For this review, take the finished solid that the model builds, in its own axes (mm). Face numbers are marked on the shaded views. A direction names the side the tool comes from. Give positions to 0.01 mm unless a question says otherwise; leave off trailing zeros. Loops run counter-clockwise (first coordinate to the right, second up) from the corner with the lowest first, then second, coordinate; pieces in that order, holes last. Notation, with made-up numbers: (32.5, -21) -> (86.5, -21) arc R33 ccw to (86.5, 8) -> close; hole circle Ø5 at (-32.75, 43). An arc over 180 degrees is marked (long way). Answer as CSV lines item,"result". Start each with the question number.
Item 1: Add section C-C on z = 2. State the section outline as (x, y) points, plus the area to 3 significant figures.
Item 2: Add section B-B on z = -51.5. State the section outline as (x, y) points, plus the area to 3 significant figures.
Item 3: For L1, parallel to Z at x = 6.3, y = 0; L2, parallel to Y at x = 2, z = -18; L3, parallel to X at y = -7, z = 8.5, list the stretches that pass through material, from the lowest coordinate up. Write a range as from..to.
Item 4: Add section A-A on x = -1.25. State the section outline as (y, z) points, plus the area to 3 significant figures.
Item 5: Machinability: for the marked faces 1 and 2, which of the approach directions +Z, -Z, +X, -X, +Y, -Y give a long, thin tool a straight path to every point of the face, cutting with its end or side? Answer none if there is none.
Item 6: The part is to be moulded in two halves that separate along X. For the marked faces 3, 4 and 5, say which applies: +X half, -X half, draft (parallel to the pull), parting line (faces both ways), or undercut.
Item 7: Clearance check with flat-ended pins moving along their axes: P1, Ø3.5, axis at x = 2, y = 3, coming from the -Z side; P2, Ø6, axis at x = -0.5, z = -47.5, coming from the +Y side; P3, Ø10, axis at y = -10, z = -10.5, coming from the +X side; P4, Ø1.5, axis at y = -9.5, z = -15, coming from the -X side. State where each tip first meets the part, or that it passes through.
```python
from build123d import *

# Parameters (mm, degrees)
SKETCH1_W           = 11.7
SKETCH1_H           = 18.2
SKETCH1_W_2         = 6.2
SKETCH1_H_2         = 15.2
BOSS_EXTRUDE1_DEPTH = 12
SKETCH4_R           = 2.55
CUT_EXTRUDE1_DEPTH  = 3
SKETCH4_3_R         = 2.55
CUT_EXTRUDE2_DEPTH  = 17.914490829
SKETCH9_W           = 11.7
SKETCH9_H           = 12
BOSS_EXTRUDE4_DEPTH = 7
SKETCH7_W           = 11.7
SKETCH7_H           = 6.6
BOSS_EXTRUDE3_DEPTH = 69
CUT_EXTRUDE4_DEPTH  = 72.812951478
FILLET1_R           = 2
FILLET2_R           = 1


# Some blends are built 0.0001 mm under size
with BuildPart() as part:
    # Sketch1 → Boss-Extrude1 (new body)
    with BuildSketch(Plane.XY):
        with Locations((1.25, 0)):
            Rectangle(SKETCH1_W, SKETCH1_H)
        Rectangle(SKETCH1_W_2, SKETCH1_H_2, mode=Mode.SUBTRACT)
    extrude(amount=BOSS_EXTRUDE1_DEPTH)

    # Sketch4 → Cut-Extrude1 (cut)
    with BuildSketch(Plane.ZY.offset(-3.1)):
        Polygon((0.515172443, 0), (3.257586221, -4.75), (8.742413779, -4.75), (11.484827557, 0), (8.742413779, 4.75), (3.257586221, 4.75), align=None)
        with Locations(Location((6, 0, 0), (0, 0, 270))):
            Circle(SKETCH4_R, mode=Mode.SUBTRACT)
    extrude(amount=-CUT_EXTRUDE1_DEPTH, mode=Mode.SUBTRACT)

    # Sketch4<3> → Cut-Extrude2 (cut, through all)
    with BuildSketch(Plane.ZY.offset(-3.1)):
        with Locations(Location((6, 0, 0), (0, 0, 270))):
            Circle(SKETCH4_3_R)
    extrude(amount=-CUT_EXTRUDE2_DEPTH, mode=Mode.SUBTRACT)

    # Sketch9 → Boss-Extrude4 (add)
    with BuildSketch(Plane.XZ.offset(9.1)):
        with Locations((1.25, 6)):
            Rectangle(SKETCH9_W, SKETCH9_H)
    extrude(amount=BOSS_EXTRUDE4_DEPTH)

    # Sketch7 → Boss-Extrude3 (add)
    with BuildSketch(Plane(origin=(0, -2.9, 0), x_dir=(1, 0, 0), z_dir=(0, 0, -1))):
        with Locations((1.25, 9.9)):
            Rectangle(SKETCH7_W, SKETCH7_H)
    extrude(amount=BOSS_EXTRUDE3_DEPTH)

    # Sketch10 → Cut-Extrude4 (cut, through all)
    with BuildSketch(Plane(origin=(7.1, 0, 0), x_dir=(0, 0, -1), z_dir=(1, 0, 0))):
        Polygon((64.5, -16.1), (64.5, -14.1), (67.5, -14.1), (67.5, -12.5), (1.5, -12.5), (1.5, -14.1), (4.5, -14.1), (4.5, -16.1), align=None)
    extrude(amount=-CUT_EXTRUDE4_DEPTH, mode=Mode.SUBTRACT)

    # Fillet1
    fillet1_edges = [part.edges().sort_by_distance(p)[0] for p in [
        (7.1, 9.1, 6),
        (-4.6, 9.1, 6),
        (-4.6, -16.1, 3.75),
        (7.1, -16.1, 3.75),
        (7.1, -9.5, -34.5),
        (-4.6, -9.5, -34.5),
        (-4.6, -16.1, -66.75),
        (7.1, -16.1, -66.75),
    ]]
    fillet(fillet1_edges, radius=FILLET1_R - 0.0001)  # a hair under: the kernel refuses the full size

    # Fillet2
    # the kernel refuses this fillet: 1 mm, written as the material it takes off along each edge
    with BuildSketch(Plane(origin=(9.6, -14.1, -4.5), x_dir=(0, -1, 0), z_dir=(-1, 0, 0)), Plane(origin=(9.6, -14.1, -64.5), x_dir=(0, 0, -1), z_dir=(-1, 0, 0))) as fillet2_piece_1:
        with BuildLine():
            CenterArc((FILLET2_R, FILLET2_R), FILLET2_R, 180, 90)
            Line((0, FILLET2_R), (0, 0))
            Line((0, 0), (FILLET2_R, 0))
        make_face()
    extrude(amount=16.7, mode=Mode.SUBTRACT)
    with BuildSketch(Plane(origin=(7.6001, -16.1, -4.5), x_dir=(0, 0, 1), z_dir=(-1, 0, 0)), Plane(origin=(7.6001, -9.5, -69), x_dir=(0, -1, 0), z_dir=(-1, 0, 0)), Plane(origin=(-5.1001, -16.1, -69), x_dir=(0, 1, 0), z_dir=(1, 0, 0)), Plane(origin=(7.6001, -16.1, -64.5), x_dir=(0, 1, 0), z_dir=(-1, 0, 0))) as fillet2_piece_2:
        with BuildLine():
            CenterArc((FILLET2_R, FILLET2_R), FILLET2_R, 180, 90)
            Line((0, FILLET2_R), (0, 0))
            Line((0, 0), (FILLET2_R, 0))
        make_face()
    extrude(amount=12.7002, mode=Mode.SUBTRACT)


solid = part.part
```
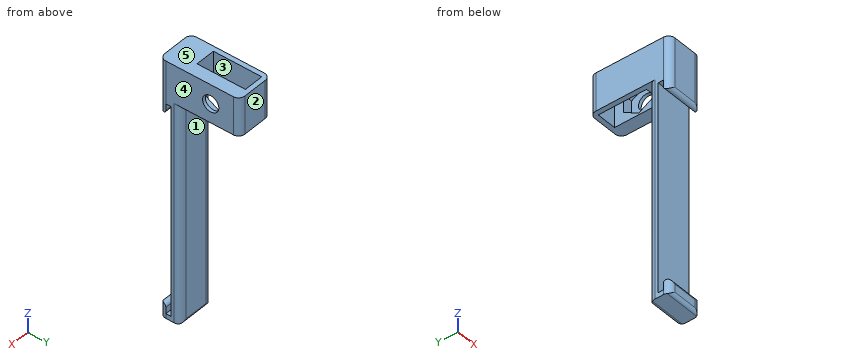
Computed values:
1,outline,"(-4.6, -14.1) arc R2 ccw to (-2.6, -16.1) -> (5.1, -16.1) arc R2 ccw to (7.1, -14.1) -> (7.1, 7.1) arc R2 ccw to (5.1, 9.1) -> (-2.6, 9.1) arc R2 ccw to (-4.6, 7.1) -> close; hole (-3.1, -7.6) -> (3.1, -7.6) -> (3.1, -2.57) -> (6.1, -2.57) -> (6.1, 2.57) -> (3.1, 2.57) -> (3.1, 7.6) -> (-3.1, 7.6) -> close"
1,area,"182 mm²"
2,outline,"(-4.6, -12.5) -> (7.1, -12.5) -> (7.1, -11.5) arc R2 ccw to (5.1, -9.5) -> (-2.6, -9.5) arc R2 ccw to (-4.6, -11.5) -> close"
2,area,"33.4 mm²"
3,L1,"0..3.45, 8.55..12"
3,L2,"-12.5..-9.5"
3,L3,"-4.6..-3.1, 3.1..7.1"
4,outline,"(-16.1, -68) arc R1 ccw to (-15.1, -69) -> (-10.5, -69) arc R1 ccw to (-9.5, -68) -> (-9.5, 0) -> (-7.6, 0) -> (-7.6, 12) -> (-16.1, 12) -> (-16.1, -3.5) arc R1 ccw to (-14.1, -3.5) -> (-14.1, -1.5) -> (-12.5, -1.5) -> (-12.5, -67.5) -> (-14.1, -67.5) -> (-14.1, -65.5) arc R1 ccw to (-16.1, -65.5) -> close; (7.6, 0) -> (9.1, 0) -> (9.1, 12) -> (7.6, 12) -> close"
4,area,"349 mm²"
5,face 1,"-Z, +X, -X, +Y"
5,face 2,"+Z, -Z, +X, -X, +Y"
6,face 3,"undercut"
6,face 4,"+X half"
6,face 5,"draft"
7,P1,"z = 0"
7,P2,"y = -9.5"
7,P3,"x = 7.1"
7,P4,"x = -4.16"
